The listing builds one solid part. Answer for the finished solid, in the listing's coordinates (mm). A direction names the side the tool comes from. Give positions to 0.01 mm unless a question says otherwise; leave off trailing zeros. Write each loop counter-clockwise with the first axis right and the second up, starting at its lowest first coordinate (ties: lowest second). Pieces come first, ordered by that corner, then holes. Notation, with made-up numbers: M 14,26 L 19,26 A14 ccw 19,44 Z; hole C -30,-26 d7. An arc over 180 degrees is marked long. Return JSON: item names as keys, results as strings.
from build123d import *

# Parameters (mm, degrees)
F0_W        = 36
F0_H        = 21.5
F0_R        = 1.625
F0_W_2      = 4
F0_H_2      = 15.5
F0_W_3      = 25
F0_H_3      = 3.5
F1_DEPTH    = 6
F2_T1_DEPTH = 6
F3_R        = 3


# Not quite as in the source:
# - a fillet or chamfer that OpenCascade refuses, or shapes differently, is made with other operations: its cross-section is extruded or revolved along the edge and cut away or added


with BuildPart() as f1:
    # F0 (on Top) → F1 (new body)
    with BuildSketch(Plane.XY):
        Rectangle(F0_W, F0_H)
        with Locations((-4.0289468229, -6.686462095)):
            Circle(F0_R, mode=Mode.SUBTRACT)
        with Locations((4.0289468229, -6.686462095)):
            Circle(F0_R, mode=Mode.SUBTRACT)
        with Locations((-14.5, 0)):
            Rectangle(F0_W_2, F0_H_2, mode=Mode.SUBTRACT)
        with Locations((14.5, 0)):
            Rectangle(F0_W_2, F0_H_2, mode=Mode.SUBTRACT)
        Polygon((-18, 10.75), (18, 10.75), (31, 10.75), (31, 23.25), (-18, 23.25), align=None)
        with Locations((15.5, 17)):
            Rectangle(F0_W_3, F0_H_3, mode=Mode.SUBTRACT)
        with Locations((-4.0289468229, -6.686462095)):
            Circle(F0_R)
        with Locations((4.0289468229, -6.686462095)):
            Circle(F0_R)
    extrude(amount=F1_DEPTH)

    # F2: fillet of radius 2 on 12 edges, made by hand

    # F2_s2 → F2_t1 (join)
    with BuildSketch(Plane.XY):
        with BuildLine():
            ThreePointArc((3, 16.75), (3.5857864376, 18.1642135624), (5, 18.75))
            Line((5, 18.75), (3, 18.75))
            Line((3, 18.75), (3, 16.75))
        make_face()
        with BuildLine():
            ThreePointArc((26, 18.75), (27.4142135624, 18.1642135624), (28, 16.75))
            Line((28, 16.75), (28, 18.75))
            Line((28, 18.75), (26, 18.75))
        make_face()
        with BuildLine():
            ThreePointArc((28, 17.25), (27.4142135624, 15.8357864376), (26, 15.25))
            Line((26, 15.25), (28, 15.25))
            Line((28, 15.25), (28, 17.25))
        make_face()
        with BuildLine():
            ThreePointArc((3, 17.25), (3.5857864376, 15.8357864376), (5, 15.25))
            Line((5, 15.25), (3, 15.25))
            Line((3, 15.25), (3, 17.25))
        make_face()
        with BuildLine():
            ThreePointArc((-14.5, -7.75), (-15.9142135624, -7.1642135624), (-16.5, -5.75))
            Line((-16.5, -5.75), (-16.5, -7.75))
            Line((-16.5, -7.75), (-14.5, -7.75))
        make_face()
        with BuildLine():
            ThreePointArc((14.5, -7.75), (13.0857864376, -7.1642135624), (12.5, -5.75))
            Line((12.5, -5.75), (12.5, -7.75))
            Line((12.5, -7.75), (14.5, -7.75))
        make_face()
        with BuildLine():
            ThreePointArc((14.5, -7.75), (15.9142135624, -7.1642135624), (16.5, -5.75))
            Line((16.5, -5.75), (16.5, -7.75))
            Line((16.5, -7.75), (14.5, -7.75))
        make_face()
        with BuildLine():
            ThreePointArc((-12.5, -5.75), (-13.0857864376, -7.1642135624), (-14.5, -7.75))
            Line((-14.5, -7.75), (-12.5, -7.75))
            Line((-12.5, -7.75), (-12.5, -5.75))
        make_face()
        with BuildLine():
            ThreePointArc((-14.5, 7.75), (-13.0857864376, 7.1642135624), (-12.5, 5.75))
            Line((-12.5, 5.75), (-12.5, 7.75))
            Line((-12.5, 7.75), (-14.5, 7.75))
        make_face()
        with BuildLine():
            ThreePointArc((-14.5, 7.75), (-15.9142135624, 7.1642135624), (-16.5, 5.75))
            Line((-16.5, 5.75), (-16.5, 7.75))
            Line((-16.5, 7.75), (-14.5, 7.75))
        make_face()
        with BuildLine():
            ThreePointArc((12.5, 5.75), (13.0857864376, 7.1642135624), (14.5, 7.75))
            Line((14.5, 7.75), (12.5, 7.75))
            Line((12.5, 7.75), (12.5, 5.75))
        make_face()
        with BuildLine():
            ThreePointArc((14.5, 7.75), (15.9142135624, 7.1642135624), (16.5, 5.75))
            Line((16.5, 5.75), (16.5, 7.75))
            Line((16.5, 7.75), (14.5, 7.75))
        make_face()
    extrude(amount=F2_T1_DEPTH)

    # F3
    f3_edges = [f1.edges().sort_by_distance(p)[0] for p in [
        (31, 10.75, 3),
        (31, 23.25, 3),
        (-18, 23.25, 3),
        (-18, -10.75, 3),
        (18, -10.75, 3),
    ]]
    fillet(f3_edges, radius=F3_R)


solid = f1.part
Item 1: A cutting plane is placed at C-C, the plane z = 2.6. Write down the section's boundary in (x, y).
Geometry results:
{"outline": "M -18,-7.75 A3 ccw -15,-10.75 L 15,-10.75 A3 ccw 18,-7.75 L 18,10.75 L 28,10.75 A3 ccw 31,13.75 L 31,20.25 A3 ccw 28,23.25 L -15,23.25 A3 ccw -18,20.25 Z; hole M -16.5,-5.75 A2 ccw -12.5,-5.75 L -12.5,5.75 A2 ccw -16.5,5.75 Z; hole M 3.02,17 A2 ccw 5,15.25 L 26,15.25 A2 ccw 27.98,17 A2 ccw 26,18.75 L 5,18.75 A2 ccw Z; hole M 12.5,-5.75 A2 ccw 16.5,-5.75 L 16.5,5.75 A2 ccw 12.5,5.75 Z"}
Item 2: A cutting plane is placed at B-B, the plane y = -4. Write down the section's boundary in (x, z), plus the area to 3 significant figures.
Geometry results:
{"outline": "M -18,0 L -16.5,0 L -16.5,6 L -18,6 Z; M -12.5,0 L 12.5,0 L 12.5,6 L -12.5,6 Z; M 16.5,0 L 18,0 L 18,6 L 16.5,6 Z", "area": "168 mm2"}
Item 3: Given pin 1 Ø3 at (y, z) = (5, 4.5) entering from +X, flat-ended and moving along its own axis, determine where the tip first touches the part or whether it passes through.
Geometry results:
{"pin 1": "stops at x = 18"}
Item 4: Determine the mould class of faces 1 (the cylindrical face through (3.662, 15.763, 2.958)), 2 (the flat face through (0, -10.75, 3)), 3 (the cylindrical face through (-17.1, 22.39, 3.04)) for opening direction X: +X half, -X half, draft (parallel to the pull), parting line (faces both ways), or undercut.
Geometry results:
{"face 1": "undercut", "face 2": "draft", "face 3": "-X half"}
Item 5: A cutting plane is placed at A-A, the plane x = 7.5. Write down the section's boundary in (y, z).
Geometry results:
{"outline": "M -10.75,0 L 15.25,0 L 15.25,6 L -10.75,6 Z; M 18.75,0 L 23.25,0 L 23.25,6 L 18.75,6 Z"}
Item 6: Which of the six approach directions +Z, -Z, +X, -X, +Y, -Y give full straight-line access (tool end or side, diameter ignored) to faces 4 (the flat face through (7, 23.25, 3)), 5 (the flat face through (23, 10.75, 3)), 6 (the cylindrical face through (27.31, 18.26, 2.96))?
Geometry results:
{"face 4": "+Z, -Z, +X, -X, +Y", "face 5": "+Z, -Z, +X, -Y", "face 6": "+Z, -Z"}
Item 7: A cutting plane is placed at D-D, the plane y = 6.5. Write down the section's boundary in (x, z), plus the area to 3 significant figures.
Geometry results:
{"outline": "M -18,0 L -16.35,0 L -16.35,6 L -18,6 Z; M -12.65,0 L 12.65,0 L 12.65,6 L -12.65,6 Z; M 16.35,0 L 18,0 L 18,6 L 16.35,6 Z", "area": "172 mm2"}
Item 8: Find the intervals of material crossed by line 1 (X direction, y = -0.5, z = 0.7); line 2 (Y direction, x = 8, z = 4.05); line 3 (Y direction, x = 22, z = 1.7), in increasing order.
Geometry results:
{"line 1": "x = -18 to -16.5, -12.5 to 12.5, 16.5 to 18", "line 2": "y = -10.75 to 15.25, 18.75 to 23.25", "line 3": "y = 10.75 to 15.25, 18.75 to 23.25"}
